Autodesk Fusion 360 part; units mm, degrees
sketch "スケッチ1" plane through (0, 0, 0) normal (0, 0, 1) x (1, 0, 0)
  line L0 (0, 0) -> (69, 0)
  line L1 (69, 0) -> (69, 23.5)
  line L2 (69, 23.5) -> (0, 23.5)
  line L3 (0, 23.5) -> (0, 0)
  circle A0 centre (55.5, 12) radius 1.75
  dimension "d1" = 12
  dimension "d2" = 3.5
  dimension "d3" = 23.5
  dimension "d4" = 69
  dimension "d5" = 13.5
extrude "押し出し1" add sketch "スケッチ1" along normal blind 28
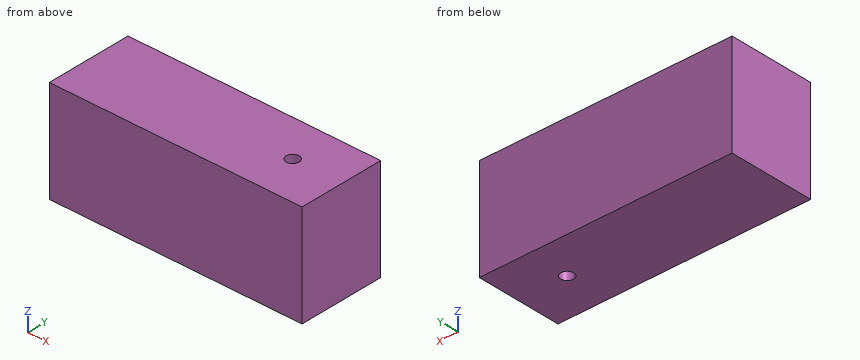
Check sheet for the modelled part. Datum: model origin and axes. Units: mm. Round coordinates to 2 decimals unless told otherwise and drop trailing zeros. Loops run counter-clockwise (first coordinate to the right, second up) from the corner with the lowest first, then second, coordinate; pieces in that order, holes last. Notation, with made-up numbers: (45, -36.5) - (72, -36.5) arc R20 ccw to (72, -25.5) - close; hole circle Ø4 at (30, 21). An arc over 180 degrees is marked (long way). Answer as a JSON object with one key per item and string values. Group by question number.
Q1. Sectioned sample at A-A, the plane y = 12. Enter the section's corners in (x, z), plus the area to 3 significant figures.
Q2. Gauge pin test, flat end, axial feed: P1, Ø1.5, axis at y = 2.5, z = 20, coming from the -X side. Record the tip position at first contact, or that the pin passes through.
Q3. Scan line: line 1 along Y through (x, z) = (55.5, 13.5). Record every from-to range of solid material in increasing order. Write a range as [from, to].
Q4. Sectioned sample at B-B, the plane x = 55.5. Enter the section's corners in (y, z), plus the area to 3 significant figures.
Solution:
{
 "1": {"outline": "(0, 0) - (53.75, 0) - (53.75, 28) - (0, 28) - close; (57.25, 0) - (69, 0) - (69, 28) - (57.25, 28) - close", "area": "1,830 mm²"},
 "2": {"P1": "stops at x = 0"},
 "3": {"line 1": "y = [0, 10.25], [13.75, 23.5]"},
 "4": {"outline": "(0, 0) - (10.25, 0) - (10.25, 28) - (0, 28) - close; (13.75, 0) - (23.5, 0) - (23.5, 28) - (13.75, 28) - close", "area": "560 mm²"}
}
